```python
from build123d import *

# Parameters (mm, degrees)
SKETCH1_W           = 57.15
SKETCH1_H           = 125.809375
SKETCH1_W_2         = 46.0375
SKETCH1_H_2         = 89.296875
BOSS_EXTRUDE1_DEPTH = 1.5875


with BuildPart() as part:
    # Sketch1 → Boss-Extrude1 (new, symmetric)
    with BuildSketch(Plane.XY):
        Rectangle(SKETCH1_W, SKETCH1_H)
        with Locations((0, -0.5953125)):
            Rectangle(SKETCH1_W_2, SKETCH1_H_2, mode=Mode.SUBTRACT)
    extrude(amount=BOSS_EXTRUDE1_DEPTH, both=True)


solid = part.part
```
The model under review builds one solid part; all positions refer to its coordinate system, in mm. A direction names the side the tool comes from. Round coordinates to 2 decimals unless told otherwise and drop trailing zeros. Write each loop counter-clockwise with the first axis right and the second up, starting at its lowest first coordinate (ties: lowest second). Pieces come first, ordered by that corner, then holes.
(1) Mouldability with a two-part tool opening along X and no side actions: class faces 1 (the flat face through (0, -45.244, 0)), 2 (the flat face through (0, -62.905, 0)), 3 (the flat face through (28.575, -1, 0)) as +X half, -X half, draft (parallel to the pull), parting line (faces both ways), or undercut.
(2) We need section A-A on x = 10. Give the boundary of the cut face in (y, z), and give its area (3 significant figures).
(3) Wall thickness on L1, parallel to Y at x = -12, z = -0.6; L2, parallel to X at y = -8.5, z = -0.2 (3 decimals): over which ranges is each line inside the solid? List them lowest first.
(4) We need section C-C on z = 1.1. Give the boundary of the cut face in (x, y) (3 decimals).
(5) We need section B-B on y = -30.5. Give the boundary of the cut face in (x, z) (1 decimal), and give its area (3 significant figures).
(6) Machinability: for faces 4 (the flat face through (-26, 1, 1.588)), 5 (the flat face through (0, 44.053, 0)), which of the approach directions +Z, -Z, +X, -X, +Y, -Y give a long, thin tool a straight path to every point of the face, cutting with its end or side? Answer none if there is none.
Findings below:
1. face 1: undercut
1. face 2: draft
1. face 3: +X half
2. outline: (-62.9, -1.59) - (-45.24, -1.59) - (-45.24, 1.59) - (-62.9, 1.59) - close; (44.05, -1.59) - (62.9, -1.59) - (62.9, 1.59) - (44.05, 1.59) - close
2. area: 116 mm2
3. L1: y = -62.9 to -45.24, 44.05 to 62.9
3. L2: x = -28.575 to -23.019, 23.019 to 28.575
4. outline: (-28.575, -62.905) - (28.575, -62.905) - (28.575, 62.905) - (-28.575, 62.905) - close; hole (-23.019, -45.244) - (23.019, -45.244) - (23.019, 44.053) - (-23.019, 44.053) - close
5. outline: (-28.6, -1.6) - (-23, -1.6) - (-23, 1.6) - (-28.6, 1.6) - close; (23, -1.6) - (28.6, -1.6) - (28.6, 1.6) - (23, 1.6) - close
5. area: 35.3 mm2
6. face 4: +Z, +X, -X, +Y, -Y
6. face 5: +Z, -Z
